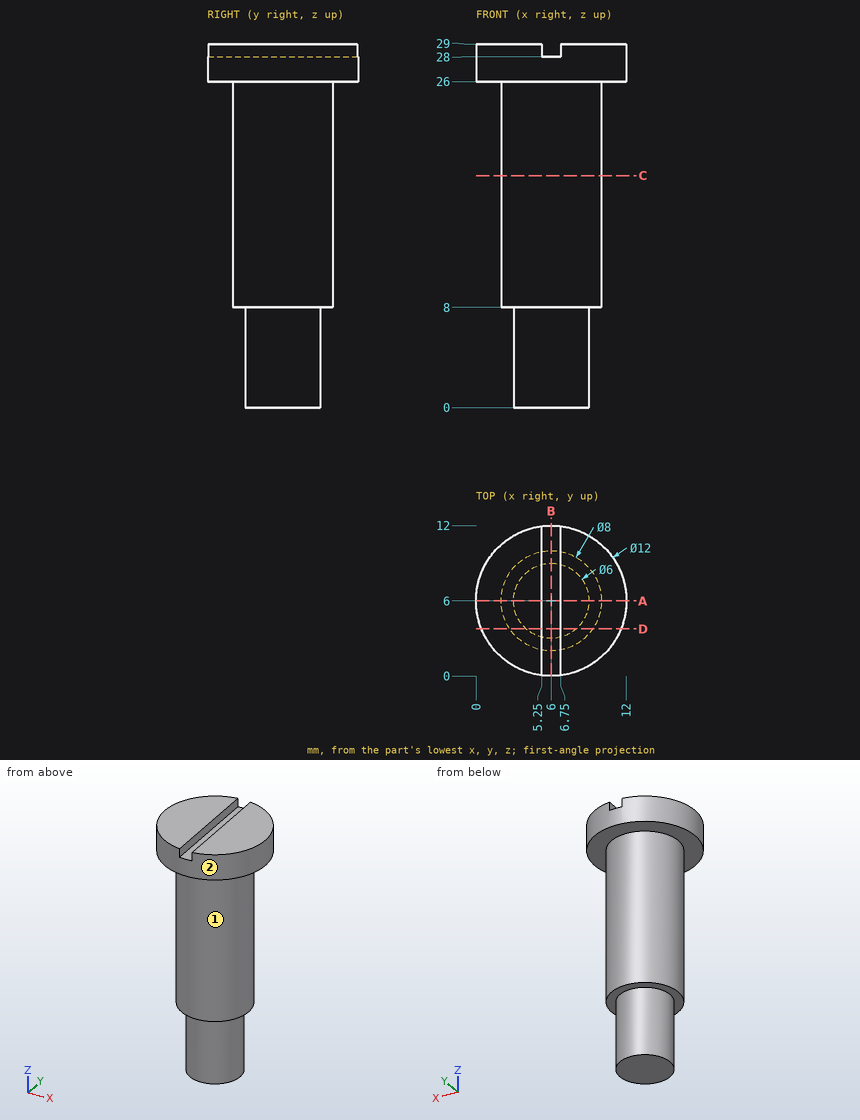
Print and shaded views of the part. All mm, measured from the part's lowest x, y and z. A direction names the side the tool comes from. Coordinates: 2 decimals unless noted, no trailing zeros. Write each loop counter-clockwise with the first axis right and the second up, starting at its lowest first coordinate (ties: lowest second). Pieces come first, ordered by that corner, then holes. Notation, with made-up numbers: (-25, -8) -> (-1, -8) arc R20 cw to (-1, 17) -> close; hole circle Ø7 at (3.5, 62). An arc over 180 degrees is marked (long way). Use CSV: the item, a comma, the result in double quotes. Start each with the question number.
Q1. 3-axis set-ups, long thin cutter, end or side, ignore diameter. For the marked faces 1 and 2: which of +Z, -Z, +X, -X, +Y, -Y reach the whole face in a straight line?
Q2. Cut at C-C, the plane z = 18.5. List the corners of the cut face in (x, y), then the cut area to 3 significant figures.
Q3. Drill centre lines: probe 1 along Z at (x, y) = (1.5, 5.75); probe 2 along Z at (x, y) = (4.5, 9.25); probe 3 along Y at (x, z) = (4.25, 10.75). Where is each one in solid material? Low to high.
Q4. Cut at D-D, the plane y = 3.75. List the corners of the cut face in (x, z).
Q5. Cut at A-A, the plane y = 6. List the corners of the cut face in (x, z), then the cut area to 4 significant figures.
Q6. Cut at B-B, the plane x = 6. List the corners of the cut face in (y, z).
Q7. Flat gauge pins, fed straight in: pin 1 Ø5 at (y, z) = (7, 21) entering from +X; pin 2 Ø1.1 at (y, z) = (4, 28.5) entering from +X; pin 3 Ø4 at (x, z) = (10.5, 15.5) entering from +Y. Where does each tip first touch, or does it go through?
Checked values:
1,face 1,"-Z"
1,face 2,"+Z, -Z"
2,outline,"circle Ø8 at (6, 6)"
2,area,"50.3 mm²"
3,probe 1,"z = 26 to 29"
3,probe 2,"z = 8 to 29"
3,probe 3,"y = 2.4 to 9.6"
4,outline,"(0.44, 26) -> (2.69, 26) -> (2.69, 8) -> (4.02, 8) -> (4.02, 0) -> (7.98, 0) -> (7.98, 8) -> (9.31, 8) -> (9.31, 26) -> (11.56, 26) -> (11.56, 29) -> (6.75, 29) -> (6.75, 28) -> (5.25, 28) -> (5.25, 29) -> (0.44, 29) -> close"
5,outline,"(0, 26) -> (2, 26) -> (2, 8) -> (3, 8) -> (3, 0) -> (9, 0) -> (9, 8) -> (10, 8) -> (10, 26) -> (12, 26) -> (12, 29) -> (6.75, 29) -> (6.75, 28) -> (5.25, 28) -> (5.25, 29) -> (0, 29) -> close"
5,area,"226.5 mm²"
6,outline,"(0, 26) -> (2, 26) -> (2, 8) -> (3, 8) -> (3, 0) -> (9, 0) -> (9, 8) -> (10, 8) -> (10, 26) -> (12, 26) -> (12, 28) -> (0, 28) -> close"
7,pin 1,"stops at x = 10"
7,pin 2,"stops at x = 11.82"
7,pin 3,"stops at y = 9.12"
